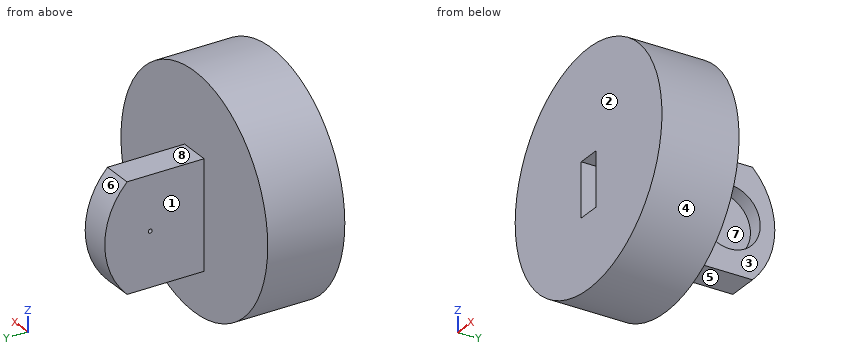
Autodesk Inventor part; units mm, degrees
ref_plane "YZ Plane" through (0, 0, 0) normal (1, 0, 0) x (0, 1, 0)
ref_plane "XZ Plane" through (0, 0, 0) normal (0, 1, 0) x (-1, 0, 0)
ref_plane "XY Plane" through (0, 0, 0) normal (0, 0, 1) x (1, 0, 0)
sketch "Sketch1" plane through (0, 0, 0) normal (0, 1, 0) x (-1, 0, 0)
  circle A0 centre (0, 0) radius 150
  dimension "d0" = 300
extrude "Extrusion1" add sketch "Sketch1" along normal blind 100
sketch "Sketch2" plane through (0, 100, 0) normal (0, 1, 0) x (1, 0, 0)
  line L0 (-20, -50) -> (20, -50)
  line L1 (20, -50) -> (20, 90)
  line L2 (20, 90) -> (-20, 90)
  line L3 (-20, 90) -> (-20, -50)
  point P0 (0, 0)
  dimension "d3" = 140
  dimension "d4" = 40
  dimension "d5" = 50
  dimension "d6" = 20
extrude "Extrusion2" add sketch "Sketch2" along normal blind 100
sketch "Sketch3" plane through (20, 100, 50) normal (1, 0, 0) x (0, 0, -1)
  line L0 (0, 100) -> (140, 100)
  arc A0 (140, 100) -> (0, 100) centre (70, 29.7912) ccw
  line L1 (0, 0) -> (0, 100)
  line L2 (0, 100) -> (140, 100)
  point P0 (50, -100)
  dimension "d9" = 99.1427
extrude "Extrusion3" add sketch "Sketch3" against normal blind 40
sketch "Sketch4" plane through (20, 100, 50) normal (1, 0, 0) x (0, 0, -1)
  circle A0 centre (70, 70) radius 40
  line L0 (200, 0) -> (-100, 0)
  line L1 (0, 0) -> (0, 100)
  point P0 (50, -100)
  dimension "d12" = 80
  dimension "d13" = 70
  dimension "d14" = 70
extrude "Extrusion4" cut sketch "Sketch4" against normal blind 20
sketch "Sketch5" plane through (0, 170, -20) normal (1, 0, 0) x (0, 0, -1)
  circle A0 centre (0, 0) radius 2.5
  circle A1 centre (0, 0) radius 40
  point P0 (-20, -170)
  dimension "d20" = 5
extrude "Extrusion5" cut sketch "Sketch5" against normal blind 20 contours A0
sketch "Sketch6" plane through (0, 0, 0) normal (0, -1, 0) x (1, 0, 0)
  line L0 (-20, 50) -> (-20, -90)
  line L1 (20, -90) -> (20, 50)
  line L2 (20, 50) -> (-20, 50)
  line L3 (-20, -90) -> (20, -90)
  line L4 (-15, 15) -> (15, 15)
  line L5 (15, 15) -> (15, -55)
  line L6 (15, -55) -> (-15, -55)
  line L7 (-15, -55) -> (-15, 15)
  point P0 (0, 0)
  point P1 (0, 15)
  point P2 (0, 50)
  point P3 (15, -20)
  point P4 (20, -20)
  dimension "d23" = 30
  dimension "d24" = 70
extrude "Extrusion6" cut sketch "Sketch6" against normal blind 90 contours L4 L5 L6 L7
sketch "Sketch7" plane through (0, 90, 0) normal (0, -1, 0) x (1, 0, 0)
  line L0 (15, -55) -> (-15, -55)
  line L1 (15, 15) -> (15, -55)
  line L2 (-15, 15) -> (15, 15)
  line L3 (-15, -55) -> (-15, 15)
  line L4 (0, 20) -> (0, -60)
  circle A0 centre (0, -20) radius 2.5
  point P0 (0, 0)
  dimension "d28" = 5
extrude "Extrusion7" cut sketch "Sketch7" against normal blind 30 contours A0 L4 | L4 A0
properties part number "Robot_arm_base"
Input: part model. Units: mm. Frame: model coordinates. Face numbers are marked on the shaded views. A direction names the side the tool comes from. Coordinates: 2 decimals unless noted, no trailing zeros. Loops run counter-clockwise (first coordinate to the right, second up) from the corner with the lowest first, then second, coordinate; pieces in that order, holes last. Notation, with made-up numbers: M 6,3.25 L 29,3.25 A23 ccw 29,42.25 Z; hole C 32.5,46 d3. An arc over 180 degrees is marked long. Answer in a Markdown table with one row per item.
1. Section B-B, the plane x = -42. Output: boundary loops of the cut face in (y, z).
Response:
| item | result |
|---|---|
| outline | M 0,-144 L 100,-144 L 100,144 L 0,144 Z |
2. First-contact query: pin 1 (4 mm diameter, centred on x = 0, z = -20, fed in from +Y); pin 2 (20 mm diameter, centred on x = 9.5, y = 155, fed in from +Z); pin 3 (12 mm diameter, centred on x = -70, z = 66, fed in from +Y). Flat tips, straight axial feed; report the tip coordinate or a pass-through.
Response:
| item | result |
|---|---|
| pin 1 | stops at y = 228.93 |
| pin 2 | stops at z = 50 |
| pin 3 | stops at y = 100 |
3. Material intervals for line 1 (Z direction, x = 0, y = 112); line 2 (Y direction, x = -11.25, z = -20); line 3 (Y direction, x = 14.25, z = -20), sorted ascending.
Response:
| item | result |
|---|---|
| line 1 | z = -90 to -22.5, -17.5 to 50 |
| line 2 | y = 90 to 167.5, 172.5 to 228.93 |
| line 3 | y = 90 to 130, 210 to 228.93 |
4. Reachability of the marked faces 1, 2, 3, 4 and 5 from +Z, -Z, +X, -X, +Y, -Y: full face, straight path, thin tool, end or side. Return the list, or none.
Response:
| item | result |
|---|---|
| face 1 | +Z, -Z, -X, +Y |
| face 2 | +Z, -Z, +X, -X, -Y |
| face 3 | +Z, -Z, +X, +Y |
| face 4 | +Y, -Y |
| face 5 | -Z, +X, -X, +Y |
5. Draft query along Y for the marked faces 6, 7 and 8. Return one class per face: pulls with the +Y half, pulls with the -Y half, needs draft (parallel to the pull), parting line crosses it, or undercut.
Response:
| item | result |
|---|---|
| face 6 | pulls with the +Y half |
| face 7 | undercut |
| face 8 | needs draft |
6. Section A-A, the plane y = 38. Output: boundary loops of the cut face in (x, z), then the cut area to 3 significant figures.
Response:
| item | result |
|---|---|
| outline | C 0,0 d300; hole M -15,-55 L 15,-55 L 15,15 L -15,15 Z |
| area | 68,600 mm2 |
7. Section C-C, the plane z = 70.5. Output: boundary loops of the cut face in (x, y).
Response:
| item | result |
|---|---|
| outline | M -132.4,0 L 132.4,0 L 132.4,100 L -132.4,100 Z |
